Geometry check sheet. Reference: drawing and pictorial views, mm from the part's lowest x, y, z. Give positions to 0.01 mm unless a question says otherwise; leave off trailing zeros. Loops run counter-clockwise (first coordinate to the right, second up) from the corner with the lowest first, then second, coordinate; pieces in that order, holes last. Notation, with made-up numbers: (59.25, 4.5) - (116.25, 4.5) arc R20 ccw to (116.25, 36.5) - close; hole circle Ø7 at (9, 60.5). An arc over 180 degrees is marked (long way). Use CSV: the item, a comma, the result in double quotes.
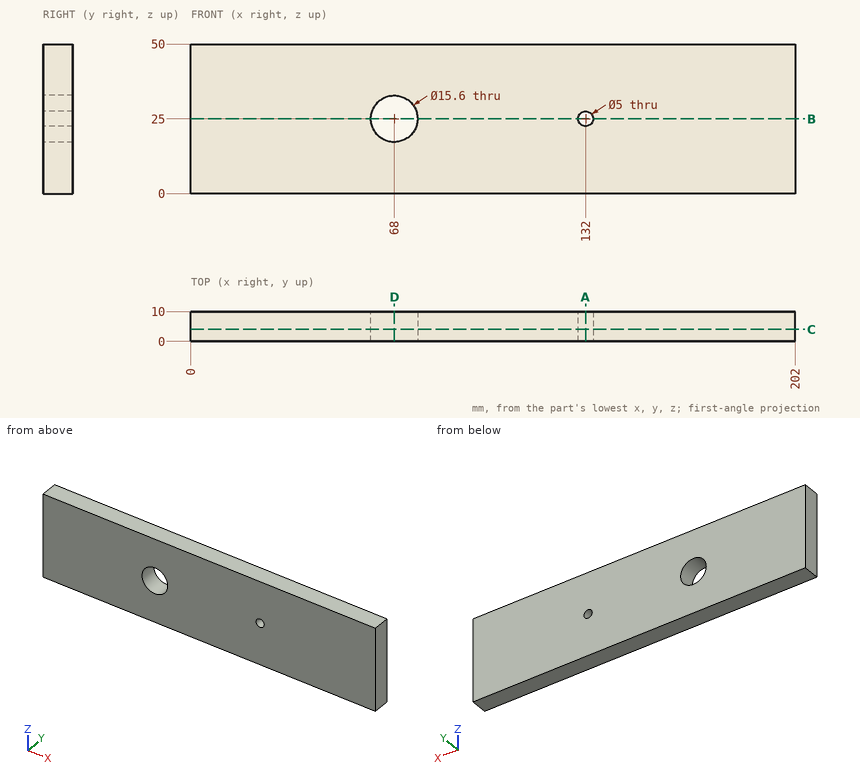
1. Scan lines: line 1 along Z through (x, y) = (68, 4.75); line 2 along Z through (x, y) = (132, 5.25); line 3 along X through (y, z) = (8.75, 26). Record each from-to range of solid material in increasing order.
Completed:
line 1,"z = 0 to 17.2, 32.8 to 50"
line 2,"z = 0 to 22.5, 27.5 to 50"
line 3,"x = 0 to 60.26, 75.74 to 129.71, 134.29 to 202"
2. Sectioned sample at D-D, the plane x = 68. Record the boundary of the cut face in (y, z), and give its area (3 significant figures).
Completed:
outline,"(0, 0) - (10, 0) - (10, 17.2) - (0, 17.2) - close; (0, 32.8) - (10, 32.8) - (10, 50) - (0, 50) - close"
area,"344 mm²"
3. Sectioned sample at A-A, the plane x = 132. Record the boundary of the cut face in (y, z).
Completed:
outline,"(0, 0) - (10, 0) - (10, 22.5) - (0, 22.5) - close; (0, 27.5) - (10, 27.5) - (10, 50) - (0, 50) - close"
4. Go/stop test with a flat-tipped pin: pin 1 Ø4.5 at (x, z) = (132, 25) entering from +Y. Record where the tip stops, or that it passes through.
Completed:
pin 1,"passes through"
5. Sectioned sample at C-C, the plane y = 4. Record the boundary of the cut face in (x, z), and give its area (3 significant figures).
Completed:
outline,"(0, 0) - (202, 0) - (202, 50) - (0, 50) - close; hole circle Ø15.6 at (68, 25); hole circle Ø5 at (132, 25)"
area,"9,890 mm²"
6. Sectioned sample at B-B, the plane z = 25. Record the boundary of the cut face in (x, y).
Completed:
outline,"(0, 0) - (60.2, 0) - (60.2, 10) - (0, 10) - close; (75.8, 0) - (129.5, 0) - (129.5, 10) - (75.8, 10) - close; (134.5, 0) - (202, 0) - (202, 10) - (134.5, 10) - close"
